```python
from build123d import *

# Parameters (mm, degrees)
F0_W     = 1524
F0_H     = 406.4
F1_DEPTH = 38.1
F2_W     = 1422.4
F2_H     = 50.8
F3_DEPTH = 63.5


with BuildPart() as f1:
    # F0 (on Top) → F1 (new body)
    with BuildSketch(Plane.XY):
        Rectangle(F0_W, F0_H)
    extrude(amount=F1_DEPTH)

    # F2 (on face) → F3 (join)
    with BuildSketch(Plane(origin=(0, 0, 0), x_dir=(1, 0, 0), z_dir=(0, 0, -1))):
        Polygon((-711.2, 152.4), (-711.2, 203.2), (-762, 203.2), (-762, -203.2), (-711.2, -203.2), (-711.2, -152.4), align=None)
        Polygon((762, -203.2), (762, 203.2), (711.2, 203.2), (711.2, 152.4), (711.2, -152.4), (711.2, -203.2), align=None)
        with Locations((0, -177.8)):
            Rectangle(F2_W, F2_H)
        with Locations((0, 177.8)):
            Rectangle(F2_W, F2_H)
    extrude(amount=F3_DEPTH)


solid = f1.part
```
Source: CAD feature listing. Evaluate the final solid. Frame: model axes, mm. A direction names the side the tool comes from. Round coordinates to 2 decimals unless told otherwise and drop trailing zeros. Write each loop counter-clockwise with the first axis right and the second up, starting at its lowest first coordinate (ties: lowest second). Pieces come first, ordered by that corner, then holes. Notation, with made-up numbers: M -29.75,54 L 22.25,54 A5 cw 22.25,58 Z; hole C 67.25,61.5 d6. An arc over 180 degrees is marked long. Answer as a JSON object with one key per item and string values. Group by question number.
(1) Section query A-A on z = -21.5. Output: boundary loops of the cut face in (x, y).
(2) Ray query, line 1 (Y direction, x = -632, z = -9); line 2 (X direction, y = -131, z = -54); line 3 (Z direction, x = -317.5, y = -8). Return the intervals inside material, ascending. Write a range as [from, to].
(3) Reachability of faces 1 (the flat face through (-10, -152.4, -31)), 2 (the flat face through (11, -203.2, -12)) from +Z, -Z, +X, -X, +Y, -Y: full face, straight path, thin tool, end or side. Return the list, or none.
(4) Section query B-B on y = 37.5. Output: boundary loops of the cut face in (x, z).
(5) Mould query, pull axis X, two halves, no side actions, for faces 3 (the flat face through (762, 3, -12)), 4 (the flat face through (711.2, -2, -31)), 5 (the flat face through (-10, 2, 0)), 6 (the flat face through (-11, 3, 38.1)). Classes: +X half, -X half, draft (parallel to the pull), parting line (faces both ways), or undercut.
(6) First-contact query: pin 1 (3 mm diameter, centred on x = -181, y = 71, fed in from -Z). Flat tip, straight axial feed; report the tip coordinate or a pass-through.
(7) Section query C-C on x = 481. Output: boundary loops of the cut face in (y, z), then the cut area to 3 significant figures.
Computed values:
{
 "1": {"outline": "M -762,-203.2 L 762,-203.2 L 762,203.2 L -762,203.2 Z; hole M -711.2,-152.4 L 711.2,-152.4 L 711.2,152.4 L -711.2,152.4 Z"},
 "2": {"line 1": "[-203.2, -152.4], [152.4, 203.2]", "line 2": "[-762, -711.2], [711.2, 762]", "line 3": "[0, 38.1]"},
 "3": {"face 1": "-Z", "face 2": "+Z, -Z, +X, -X, -Y"},
 "4": {"outline": "M -762,-63.5 L -711.2,-63.5 L -711.2,0 L 711.2,0 L 711.2,-63.5 L 762,-63.5 L 762,38.1 L -762,38.1 Z"},
 "5": {"face 3": "+X half", "face 4": "undercut", "face 5": "undercut", "face 6": "draft"},
 "6": {"pin 1": "z = 0"},
 "7": {"outline": "M -203.2,-63.5 L -152.4,-63.5 L -152.4,0 L 152.4,0 L 152.4,-63.5 L 203.2,-63.5 L 203.2,38.1 L -203.2,38.1 Z", "area": "21,900 mm^2"}
}
